Could you check a few things on this drawing? It's one solid part, dimensions in mm from its lowest x, y, z. A direction names the side the tool comes from. Coordinates: 2 decimals unless noted, no trailing zeros. Order: outer loops, then holes, each group sorted by start corner. A loop starts at its lowest first (then second) coordinate and runs counter-clockwise, first axis right, second up.
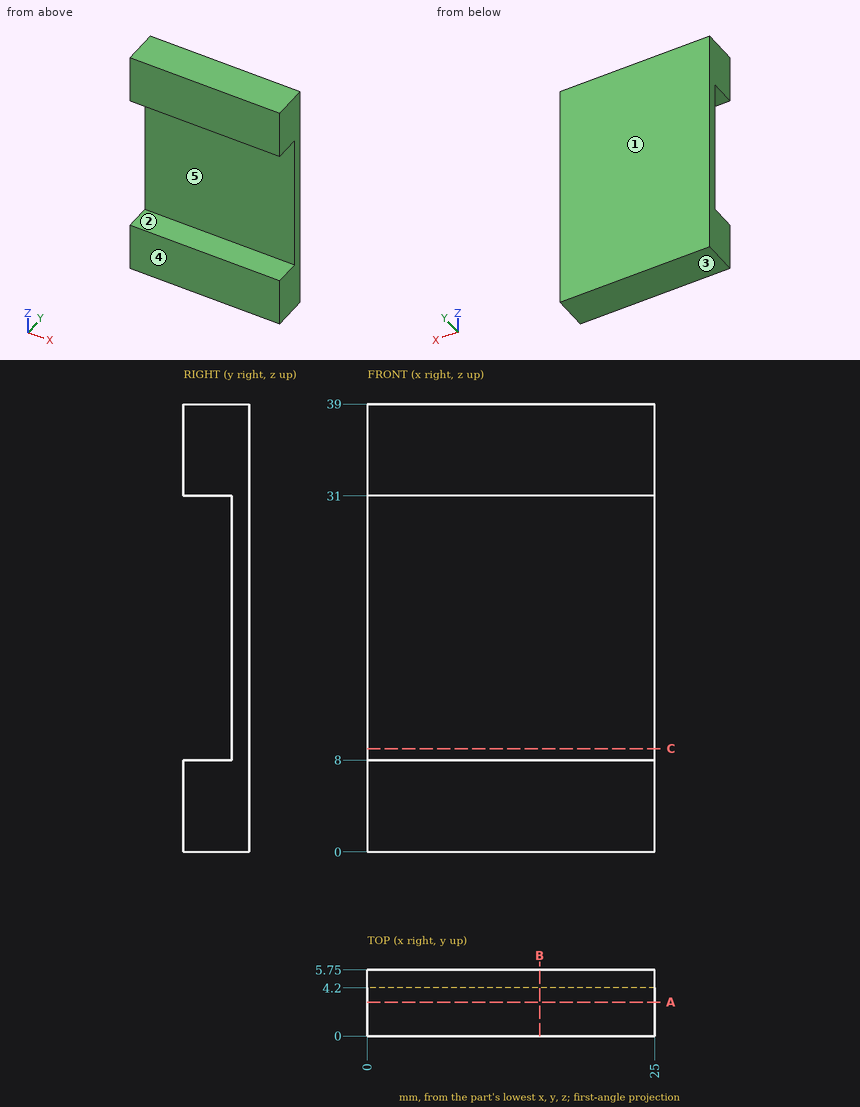
1. Please list where these lines run through material, in increasing order: probe 1 along Z at (x, y) = (20.75, 1.9); probe 2 along Y at (x, z) = (20.75, 9).
Completed:
probe 1: z = 0 to 8, 31 to 39
probe 2: y = 4.2 to 5.75
2. Imagine slicing it at B-B on x = 15. Please give me the cut outline in (y, z), then the cut area to 3 significant figures.
Completed:
outline: (0, 0) - (5.75, 0) - (5.75, 39) - (0, 39) - (0, 31) - (4.2, 31) - (4.2, 8) - (0, 8) - close
area: 128 mm2
3. Thinking about a two-plate mould opening in Z: for the marked faces 1, 2 and 3, which applies, pulls with the +Z half, pulls with the -Z half, needs draft (parallel to the pull), parting line crosses it, or undercut?
Completed:
face 1: needs draft
face 2: undercut
face 3: pulls with the -Z half
4. Imagine slicing it at C-C on z = 9. Please give me the cut outline in (x, y).
Completed:
outline: (0, 4.2) - (25, 4.2) - (25, 5.75) - (0, 5.75) - close
5. Imagine slicing it at A-A on y = 2.95. Please give me the cut outline in (x, z), then the cut area to 3 significant figures.
Completed:
outline: (0, 0) - (25, 0) - (25, 8) - (0, 8) - close; (0, 31) - (25, 31) - (25, 39) - (0, 39) - close
area: 400 mm2
6. I'm going to push a flat-ended pin straight in: pin 1 (1.5 mm diameter, centred on x = 14, z = 9, fed in from -Y). Where does the tip first touch, or does it pass through?
Completed:
pin 1: stops at y = 4.2
7. On a 3-axis mill with a long thin cutter (end or side, diameter ignored), from which of +Z, -Z, +X, -X, +Y, -Y can I reach the whole of each face in a straight line? I mean the marked faces 4 and 5. Say none if no direction works.
Completed:
face 4: +Z, -Z, +X, -X, -Y
face 5: +X, -X, -Y
